Check sheet for the drawn part. Datum: minimum x, y, z corner. Units: mm. A direction names the side the tool comes from. Coordinates: 2 decimals unless noted, no trailing zeros. Write each loop counter-clockwise with the first axis right and the second up, starting at its lowest first coordinate (ties: lowest second). Pieces come first, ordered by that corner, then holes. Notation, with made-up numbers: (63.25, -31.5) - (103.25, -31.5) arc R37 ccw to (103.25, 5.5) - close; hole circle Ø8 at (47.25, 38.5). An arc over 180 degrees is marked (long way). Use one line per item in the form item = value. Start each with the question number.
1. Cross-section at D-D on y = 10. Record the boundary of the cut face in (x, z).
2. Tool access check on the marked faces 1 and 2. Record the directions out of +Z, -Z, +X, -X, +Y, -Y that give a thin tool (end or side, any length) a straight path to the whole face; none if there is none.
3. Cross-section at A-A on z = 2. Record the boundary of the cut face in (x, y) (1 decimal).
4. Cross-section at B-B on x = 2. Give the number of separate pieces and of enclosed holes in the cut face.
5. Go/stop test with flat-tipped pins: pin 1 Ø2.5 at (x, y) = (3.18, 10.64) entering from -Z; pin 2 Ø5 at (x, y) = (9.52, 10.64) entering from -Z; pin 3 Ø4.5 at (x, y) = (11, 11) entering from -Z (1 decimal). Record where each tip stops, or that it passes through.
6. Scan lines: line 1 along Y through (x, z) = (9.75, 1.5) (1 decimal); line 2 along X through (y, z) = (9.75, 3.5); line 3 along Y through (x, z) = (2, 2.5) (1 decimal). Record each from-to range of solid material in increasing order.
7. Draft check along Y on the marked faces 3, 4, 5 and 6. Enter one of: +Y half, -Y half, draft (parallel to the pull), parting line (faces both ways), or undercut.
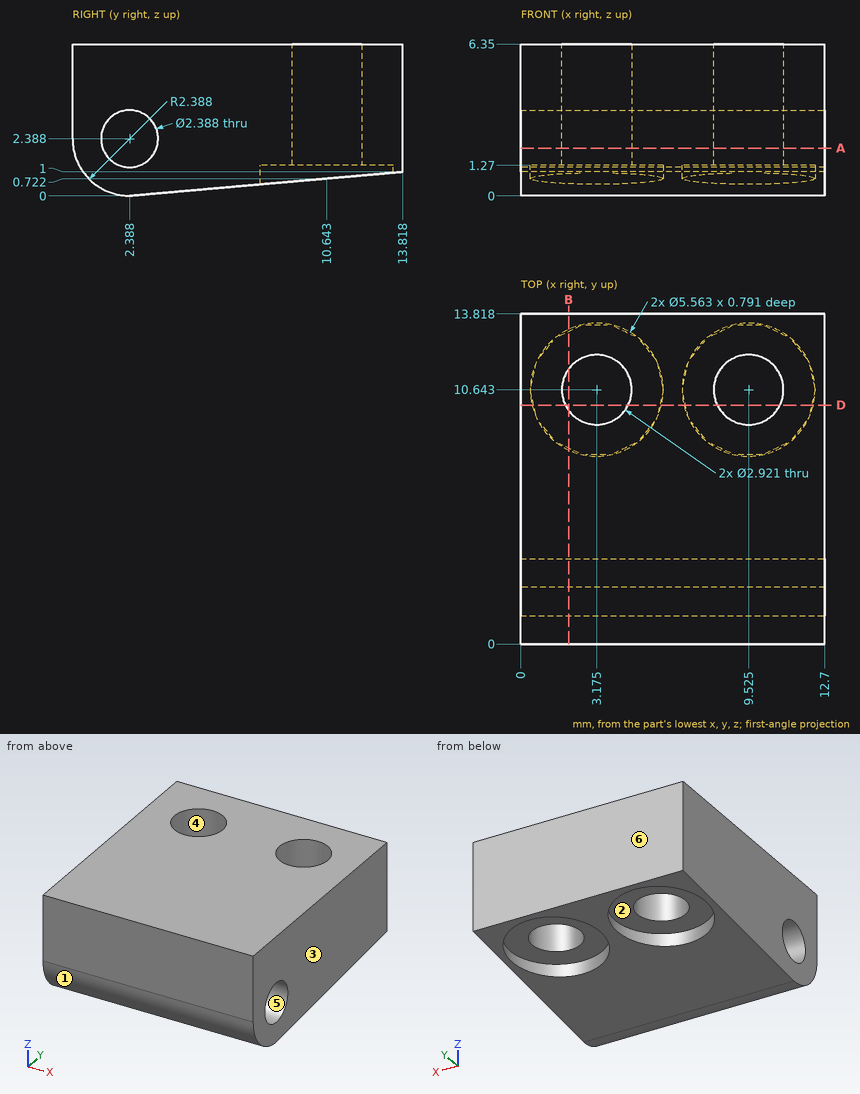
Final values:
q1.outline = (0, 0.67) - (0.47, 0.67) - (0.47, 1.27) - (1.86, 1.27) - (1.86, 6.35) - (0, 6.35) - close; (4.49, 1.27) - (5.88, 1.27) - (5.88, 0.67) - (6.82, 0.67) - (6.82, 1.27) - (8.21, 1.27) - (8.21, 6.35) - (4.49, 6.35) - close; (10.84, 1.27) - (12.23, 1.27) - (12.23, 0.67) - (12.7, 0.67) - (12.7, 6.35) - (10.84, 6.35) - close
q2.face_1 = -Z, +X, -X, -Y
q2.face_2 = -Z
q3.outline = (0, 0) - (12.7, 0) - (12.7, 1.3) - (0, 1.3) - close; (0, 3.5) - (12.7, 3.5) - (12.7, 13.8) - (0, 13.8) - close; hole circle Ø2.9 at (3.2, 10.6); hole circle Ø2.9 at (9.5, 10.6)
q4.separate_pieces = 2
q4.enclosed_holes = 1
q5.pin_1 = through
q5.pin_2 = 1.27
q5.pin_3 = 0.6
q6.line_1 = 0.2 to 1.6, 3.2 to 9.2, 12.1 to 13.8
q6.line_2 = 0 to 2.02, 4.33 to 8.37, 10.68 to 12.7
q6.line_3 = 0 to 1.2, 3.6 to 9.8, 11.5 to 13.8
q7.face_3 = draft
q7.face_4 = undercut
q7.face_5 = undercut
q7.face_6 = +Y half
